The model under review builds one solid part; all positions refer to its coordinate system, in mm. A direction names the side the tool comes from. Round coordinates to 2 decimals unless told otherwise and drop trailing zeros. Loops run counter-clockwise (first coordinate to the right, second up) from the corner with the lowest first, then second, coordinate; pieces in that order, holes last. Notation, with made-up numbers: M -32.75,32 L -23.75,32 A28 ccw -23.75,52 Z; hole C -11.5,-10 d9. An arc over 180 degrees is marked long. Return JSON: item names as keys, results as strings. Group by question number.
Q1. Consider section A-A (y = -0.5). State the section outline as (x, z) points.
Q2. For faces 1 (the face through (3.6, 1.819, 12.5)), 2 (the face through (3.9, 1.819, -2.5)), 3 (the face through (-6.293, -11, 5)), 4 (the face through (-9, -10.181, 5)), 5 (the face through (21.665, -3.519, 1.095)), list the 3-axis set-ups (+Z, -Z, +X, -X, +Y, -Y) from which the entire face can be reached by the end or side of a thin tool; tool diameter is ignored.
Q3. Consider section C-C (z = 5). State the section outline as (x, y) points, and give its area (3 significant figures).
Q4. Clearance check with flat-ended pins moving along their axes: pin 1 Ø3 at (y, z) = (1, 6) entering from -X; pin 2 Ø6 at (x, y) = (-14, 1.5) entering from +Z; pin 3 Ø2.5 at (x, z) = (16.5, 2.5) entering from -Y. State where each tip first meets the part, or that it passes through.
Q5. To check wall thickness, follow line 1 along X through (y, z) = (-5, 4.25); line 2 along X through (y, z) = (-10.75, -1.5); line 3 along Y through (x, z) = (-8, 6.25). State the ranges of each line that lie inside material, in increasing order.
Q6. Draft analysis for pull direction X (two halves, no side actions). For faces 6 (the face through (4, -5, -5)), 7 (the face through (13.782, -5, -2)), 8 (the face through (-14.251, 1.285, 4.479)), state which applies: pulls with the +X half, pulls with the -X half, needs draft (parallel to the pull), parting line crosses it, or undercut.
Q7. Consider section D-D (x = -5.5). State the section outline as (y, z) points.
Q8. Consider section B-B (y = 3.5). State the section outline as (x, z) points.
from build123d import *

# Parameters (mm, degrees)
SKETCH1_W            = 30
SKETCH1_H            = 15
BOSS_EXTRUDE1_DEPTH  = 10
SKETCH2_W            = 20
SKETCH2_H            = 14
BOSS_EXTRUDE2_DEPTH  = 5
SKETCH3_W            = 20.074773711
SKETCH3_H            = 14
BOSS_EXTRUDE3_DEPTH  = 5
SKETCH4_W            = 20
SKETCH4_H            = 10
BOSS_EXTRUDE4_DEPTH  = 2
SKETCH5_R            = 4
BOSS_EXTRUDE6_DEPTH  = 6
SKETCH6_R            = 4
BOSS_EXTRUDE7_DEPTH  = 6
SKETCH8_R            = 1.5
BOSS_EXTRUDE9_DEPTH  = 5
SKETCH10_R           = 1.5
BOSS_EXTRUDE10_DEPTH = 5


with BuildPart() as part:
    # Sketch1 → Boss-Extrude1 (new body)
    with BuildSketch(Plane.XY):
        with Locations((3.707224335, -2.680608365)):
            Rectangle(SKETCH1_W, SKETCH1_H)
    extrude(amount=BOSS_EXTRUDE1_DEPTH)

    # Sketch2 → Boss-Extrude2 (add)
    with BuildSketch(Plane.XY.offset(10)):
        with Locations((3.707224335, -5.180608365)):
            Rectangle(SKETCH2_W, SKETCH2_H)
    extrude(amount=BOSS_EXTRUDE2_DEPTH)

    # Sketch3 → Boss-Extrude3 (add)
    with BuildSketch(Plane(origin=(0, 0, 0), x_dir=(-1, 0, 0), z_dir=(0, 0, -1))):
        with Locations((-3.74461119, -5.180608365)):
            Rectangle(SKETCH3_W, SKETCH3_H)
    extrude(amount=BOSS_EXTRUDE3_DEPTH)

    # Sketch4 → Boss-Extrude4 (add)
    with BuildSketch(Plane.XZ.offset(10.180608365)):
        with Locations((3.707224335, 5)):
            Rectangle(SKETCH4_W, SKETCH4_H)
    extrude(amount=BOSS_EXTRUDE4_DEPTH)

    # Sketch5 → Boss-Extrude6 (add)
    with BuildSketch(Plane(origin=(18.707224335, 0, 0), x_dir=(0, 0, -1), z_dir=(1, 0, 0))):
        with Locations(Location((-5, -2.651445807, 0), (0, 0, 90))):
            Circle(SKETCH5_R)
    extrude(amount=BOSS_EXTRUDE6_DEPTH)

    # Sketch6 → Boss-Extrude7 (add)
    with BuildSketch(Plane.ZY.offset(11.292775665)):
        with Locations((5, -2.680608365)):
            Circle(SKETCH6_R)
    extrude(amount=BOSS_EXTRUDE7_DEPTH)

    # Sketch8 → Boss-Extrude9 (add)
    with BuildSketch(Plane.ZY.offset(17.292775665)):
        with Locations((5, -2.680608365)):
            Circle(SKETCH8_R)
    extrude(amount=BOSS_EXTRUDE9_DEPTH)

    # Sketch10 → Boss-Extrude10 (add)
    with BuildSketch(Plane(origin=(24.707224335, 0, 0), x_dir=(0, 0, -1), z_dir=(1, 0, 0))):
        with Locations(Location((-5, -2.651445807, 0), (0, 0, 90))):
            Circle(SKETCH10_R)
    extrude(amount=BOSS_EXTRUDE10_DEPTH)

    # Sketch9 → Revolve3 (revolve)
    with BuildSketch(Plane.ZY.offset(22.292775665)):
        with BuildLine():
            Line((5, 2.348554193), (5, -7.651445807))
            ThreePointArc((5, -7.651445807), (0, -2.651445807), (5, 2.348554193))
        make_face()
    revolve(axis=Axis((-22.292775665, 2.348554193, 5), (0, -1, 0)))

    # Sketch11 → Revolve4 (revolve)
    with BuildSketch(Plane(origin=(29.707224335, 0, 0), x_dir=(0, 0, -1), z_dir=(1, 0, 0))):
        with BuildLine():
            Line((-5, 2.348554193), (-5, -7.651445807))
            ThreePointArc((-5, -7.651445807), (-10, -2.651445807), (-5, 2.348554193))
        make_face()
    revolve(axis=Axis((29.707224335, 2.348554193, 5), (0, -1, 0)))

    # Sketch7 → Cut-Revolve2 (revolve, cut)
    with BuildSketch(Plane(origin=(0, 4.819391635, 0), x_dir=(1, 0, 0), z_dir=(0, 1, 0))):
        with BuildLine():
            Line((3.707224335, 2.5), (3.707224335, -12.5))
            ThreePointArc((3.707224335, -12.5), (-3.792775665, -5), (3.707224335, 2.5))
        make_face()
    revolve(axis=Axis((3.707224335, 4.819391635, -2.5), (0, 0, 1)), mode=Mode.SUBTRACT)


solid = part.part
Values:
{
 "1": {"outline": "C -22.29,5 d9.03; M -17.29,1.65 L -11.29,1.65 L -11.29,0 L -6.29,0 L -6.29,-5 L 13.78,-5 L 13.78,0 L 18.71,0 L 18.71,1.63 L 24.71,1.63 L 24.71,8.37 L 18.71,8.37 L 18.71,10 L 13.71,10 L 13.71,15 L -6.29,15 L -6.29,10 L -11.29,10 L -11.29,8.35 L -17.29,8.35 Z; C 29.71,5 d9.03; hole C 3.71,5 d10.57"},
 "2": {"face 1": "+Z, +X, -X, +Y", "face 2": "-Z, +X, -X, +Y", "face 3": "-X, -Y", "face 4": "+Z, -Z, -X, -Y", "face 5": "none"},
 "3": {"outline": "M -17.53,-4.18 L -17.29,-4.18 L -17.29,-6.68 L -11.29,-6.68 L -11.29,-10.18 L -6.29,-10.18 L -6.29,-12.18 L 13.71,-12.18 L 13.71,-10.18 L 18.71,-10.18 L 18.71,-6.65 L 24.71,-6.65 L 24.71,-4.15 L 24.94,-4.15 A5 ccw long 24.94,-1.15 L 24.71,-1.15 L 24.71,1.35 L 18.71,1.35 L 18.71,4.82 L 11.21,4.82 A7.5 cw -3.79,4.82 L -11.29,4.82 L -11.29,1.32 L -17.29,1.32 L -17.29,-1.18 L -17.51,-1.18 A5 ccw long Z", "area": "655 mm2"},
 "4": {"pin 1": "stops at x = -26.74", "pin 2": "stops at z = 10", "pin 3": "stops at y = -10.18"},
 "5": {"line 1": "x = -26.64 to -17.94, -17.29 to 24.71, 25.36 to 34.06", "line 2": "x = -6.29 to 13.78", "line 3": "y = -10.18 to 4.82"},
 "6": {"face 6": "needs draft", "face 7": "pulls with the +X half", "face 8": "undercut"},
 "7": {"outline": "M -12.18,-5 L 1.82,-5 L 1.82,0 L 4.82,0 L 4.82,10 L 1.82,10 L 1.82,15 L -12.18,15 Z"},
 "8": {"outline": "M -11.29,0 L -1.73,0 A7.38 cw -1.73,10 L -11.29,10 Z; M 9.14,0 L 18.71,0 L 18.71,10 L 9.14,10 A7.38 cw Z"}
}
